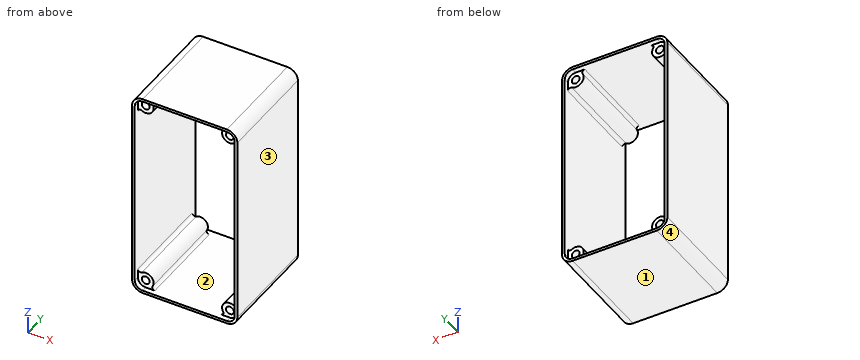
from build123d import *

# Parameters (mm, degrees)
ESQUISSE1_R             = 0.7500000000000007
BOSS_EXTRU_1_DEPTH      = 19.5
ENL_V_START             = -1
ESQUISSE2_R             = 1.5000000000042053
ESQUISSE2_R_2           = 1.5000000000000118
ESQUISSE2_R_3           = 1.5000000000000042
ESQUISSE2_R_4           = 1.4999999999999973
ENL_V_MAT_EXTRU_1_DEPTH = 1
ENL_V_START_2           = -19.5
ESQUISSE2_2_R           = 1.5000000000042053
ESQUISSE2_2_R_2         = 1.5000000000000118
ESQUISSE2_2_R_3         = 1.5000000000000042
ESQUISSE2_2_R_4         = 1.4999999999999973
ENL_V_MAT_EXTRU_2_DEPTH = 1
CONG_1_R                = 0.5
CONG_2_START            = -18.5
CONG_2_DEPTH            = 17.5


with BuildPart() as part:
    # Esquisse1 → Boss.-Extru.1 (new body)
    with BuildSketch(Plane.XZ.offset(19.5)):
        with BuildLine():
            Line((-55.9111281070707, 24.325812619498315), (-39.91112810707456, 24.325812619498663))
            ThreePointArc((-39.91112810707456, 24.325812619498663), (-38.49691454470147, 24.911599057125567), (-37.91112810707456, 26.325812619498663))
            Line((-37.91112810707456, 26.325812619498663), (-37.91112810707456, 62.32581261950286))
            ThreePointArc((-37.91112810707456, 62.32581261950286), (-38.49691454470147, 63.740026181875955), (-39.91112810707456, 64.32581261950286))
            Line((-39.91112810707456, 64.32581261950286), (-55.91112810707387, 64.32581261950355))
            ThreePointArc((-55.91112810707387, 64.32581261950355), (-57.3253416694479, 63.74002618187669), (-57.91112810707526, 62.32581261950286))
            Line((-57.91112810707526, 62.32581261950286), (-57.91112810707456, 26.325812619502862))
            ThreePointArc((-57.91112810707456, 26.325812619502862), (-57.325341669446544, 24.911599057126917), (-55.9111281070707, 24.325812619498315))
        make_face()
        with Locations(Location((-39.91112810707456, 26.325812619498663, 0), (0, 0, 90))):
            Circle(ESQUISSE1_R, mode=Mode.SUBTRACT)
        with Locations(Location((-39.91112810707456, 62.32581261950286, 0), (0, 0, 90))):
            Circle(ESQUISSE1_R, mode=Mode.SUBTRACT)
        with Locations(Location((-55.91112810707456, 62.32581261950286, 0), (0, 0, 90))):
            Circle(ESQUISSE1_R, mode=Mode.SUBTRACT)
        with Locations(Location((-55.911128107070354, 26.325812619502862, 0), (0, 0, 90))):
            Circle(ESQUISSE1_R, mode=Mode.SUBTRACT)
        with BuildLine():
            Line((-38.41112810707456, 62.32581261950286), (-38.41112810707455, 26.325812619498663))
            ThreePointArc((-38.41112810707455, 26.325812619498663), (-40.97178827885439, 27.38647279127849), (-39.91112810707456, 24.825812619498656))
            Line((-39.91112810707456, 24.825812619498656), (-55.911128107070354, 24.825812619498652))
            ThreePointArc((-55.911128107070354, 24.825812619498652), (-54.850467935287554, 27.386472791285662), (-57.41112810707456, 26.325812619502862))
            Line((-57.41112810707456, 26.325812619502862), (-57.41112810707456, 62.32581261950286))
            ThreePointArc((-57.41112810707456, 62.32581261950286), (-54.85046793529474, 61.26515244772304), (-55.91112810707456, 63.82581261950286))
            Line((-55.91112810707456, 63.82581261950286), (-39.91112810707456, 63.82581261950286))
            ThreePointArc((-39.91112810707456, 63.82581261950286), (-40.97178827885438, 61.26515244772304), (-38.41112810707456, 62.32581261950286))
        make_face(mode=Mode.SUBTRACT)
    extrude(amount=-BOSS_EXTRU_1_DEPTH)

    # Esquisse2 → Enlèv. mat.-Extru.1 (cut)
    with BuildSketch(Plane(origin=(0, 0, 0), x_dir=(1, 0, 0), z_dir=(0, 1, 0)).offset(ENL_V_START)):
        with Locations((-55.911128107070354, -26.325812619502862)):
            Circle(ESQUISSE2_R)
        with Locations((-39.91112810707456, -26.325812619498663)):
            Circle(ESQUISSE2_R_2)
        with Locations((-55.91112810707456, -62.32581261950286)):
            Circle(ESQUISSE2_R_3)
        with Locations((-39.91112810707456, -62.32581261950286)):
            Circle(ESQUISSE2_R_4)
    extrude(amount=ENL_V_MAT_EXTRU_1_DEPTH, mode=Mode.SUBTRACT)

    # Esquisse2<2> → Enlèv. mat.-Extru.2 (cut)
    with BuildSketch(Plane(origin=(0, 0, 0), x_dir=(1, 0, 0), z_dir=(0, 1, 0)).offset(ENL_V_START_2)):
        with Locations((-55.911128107070354, -26.325812619502862)):
            Circle(ESQUISSE2_2_R)
        with Locations((-39.91112810707456, -26.325812619498663)):
            Circle(ESQUISSE2_2_R_2)
        with Locations((-55.91112810707456, -62.32581261950286)):
            Circle(ESQUISSE2_2_R_3)
        with Locations((-39.91112810707456, -62.32581261950286)):
            Circle(ESQUISSE2_2_R_4)
    extrude(amount=ENL_V_MAT_EXTRU_2_DEPTH, mode=Mode.SUBTRACT)

    # Congé1
    cong_1_edges = [part.edges().sort_by_distance(p)[0] for p in [
        (-57.41112810707456, -9.75, 26.325812619502862),
        (-38.41112810707456, -9.75, 26.325812619498663),
        (-57.41112810707456, -9.75, 62.32581261950286),
        (-38.41112810707456, -9.75, 62.32581261950286),
    ]]
    fillet(cong_1_edges, radius=CONG_1_R - 0.0001)  # a hair under: the kernel refuses the full size

    # Congé2: read off the stored shape, not the designer's step
    # Congé2 outline → Congé2 (add)
    with BuildSketch(Plane(origin=(0, 0, 0), x_dir=(1, 0, 0), z_dir=(0, 1, 0)).offset(CONG_2_START)):
        with BuildLine():
            ThreePointArc((-39.911128107, -63.82581262), (-40.661128107, -63.624850726), (-41.210166213, -63.07581262))
            ThreePointArc((-41.210166213, -63.07581262), (-41.210166213, -63.57581262), (-41.643178915, -63.82581262))
            Line((-41.643178915, -63.82581262), (-39.911128107, -63.82581262))
        make_face()
        with BuildLine():
            Line((-55.911128107, -63.82581262), (-54.1790773, -63.82581262))
            ThreePointArc((-54.1790773, -63.82581262), (-54.612090001, -63.57581262), (-54.612090001, -63.07581262))
            ThreePointArc((-54.612090001, -63.07581262), (-55.161128107, -63.624850725), (-55.911128107, -63.82581262))
        make_face()
        with BuildLine():
            Line((-39.911128107, -24.825812619), (-41.643178915, -24.825812619))
            ThreePointArc((-41.643178915, -24.825812619), (-41.210166213, -25.075812619), (-41.210166213, -25.575812619))
            ThreePointArc((-41.210166213, -25.575812619), (-40.661128107, -25.026774513), (-39.911128107, -24.825812619))
        make_face()
        with BuildLine():
            ThreePointArc((-54.612090001, -25.575812619), (-54.612090001, -25.075812619), (-54.179077299, -24.825812619))
            Line((-54.179077299, -24.825812619), (-55.911128107, -24.825812619))
            ThreePointArc((-55.911128107, -24.825812619), (-55.161128107, -25.026774514), (-54.612090001, -25.575812619))
        make_face()
    extrude(amount=CONG_2_DEPTH)


solid = part.part
For this review, take the finished solid that the model builds, in its own axes (mm). Face numbers are marked on the shaded views. Give positions to 0.01 mm unless a question says otherwise; leave off trailing zeros. Loops run counter-clockwise (first coordinate to the right, second up) from the corner with the lowest first, then second, coordinate; pieces in that order, holes last.
Item 1: Take a section at A-A, the plane x = -52. State the section outline as (y, z) points, and give its area (3 significant figures).
Item 2: Draft analysis for pull direction X (two halves, no side actions). For the marked faces 1, 2, 3 and 4, state which applies: +X half, -X half, draft (parallel to the pull), parting line (faces both ways), or undercut.
Item 3: Take a section at B-B, the plane z = 48. State the section outline as (x, y) points, and give its area (3 significant figures).
Item 4: For line 1 along X through (y, z) = (-6.5, 48); line 2 along Z through (x, y) = (-51, -6.5); line 3 along Z through (x, y) = (-56, -12.75), list the stretches that pass through material, from the lowest coordinate up.
Item 5: Insertion check: pin 1 (1 mm diameter, centred on x = -56, z = 62.5, fed in from -Y); pin 2 (1.7 mm diameter, centred on x = -55.91, z = 62.33, fed in from -Y); pin 3 (1 mm diameter, centred on x = -40.5, z = 62.5, fed in from +Y). Each pin has a flat end and moves straight along its axis. Give the tip position at first contact, or say it passes through.
Item 6: Take a section at C-C, the plane y = -13.25. Give the number of separate pieces and of enclosed holes in the cut face, and give its area (3 significant figures).
Calculated:
1. outline: (-19.5, 24.33) - (0, 24.33) - (0, 24.83) - (-19.5, 24.83) - close; (-19.5, 63.83) - (0, 63.83) - (0, 64.33) - (-19.5, 64.33) - close
1. area: 19.5 mm2
2. face 1: draft
2. face 2: undercut
2. face 3: +X half
2. face 4: -X half
3. outline: (-57.91, -19.5) - (-57.41, -19.5) - (-57.41, 0) - (-57.91, 0) - close; (-38.41, -19.5) - (-37.91, -19.5) - (-37.91, 0) - (-38.41, 0) - close
3. area: 19.5 mm2
4. line 1: x = -57.91 to -57.41, -38.41 to -37.91
4. line 2: z = 24.33 to 24.83, 63.83 to 64.33
4. line 3: z = 24.33 to 25.58, 27.07 to 27.82, 60.83 to 61.58, 63.07 to 64.32
5. pin 1: passes through
5. pin 2: stops at y = -18.5
5. pin 3: stops at y = -1
6. separate pieces: 1
6. enclosed holes: 5
6. area: 81.0 mm2
